Could you check a few things on this drawing? It's one solid part, dimensions in mm from its lowest x, y, z. Give positions to 0.01 mm unless a question says otherwise; leave off trailing zeros. Order: outer loops, then holes, each group sorted by start corner. A loop starts at its lowest first (then second) coordinate and runs counter-clockwise, first axis right, second up.
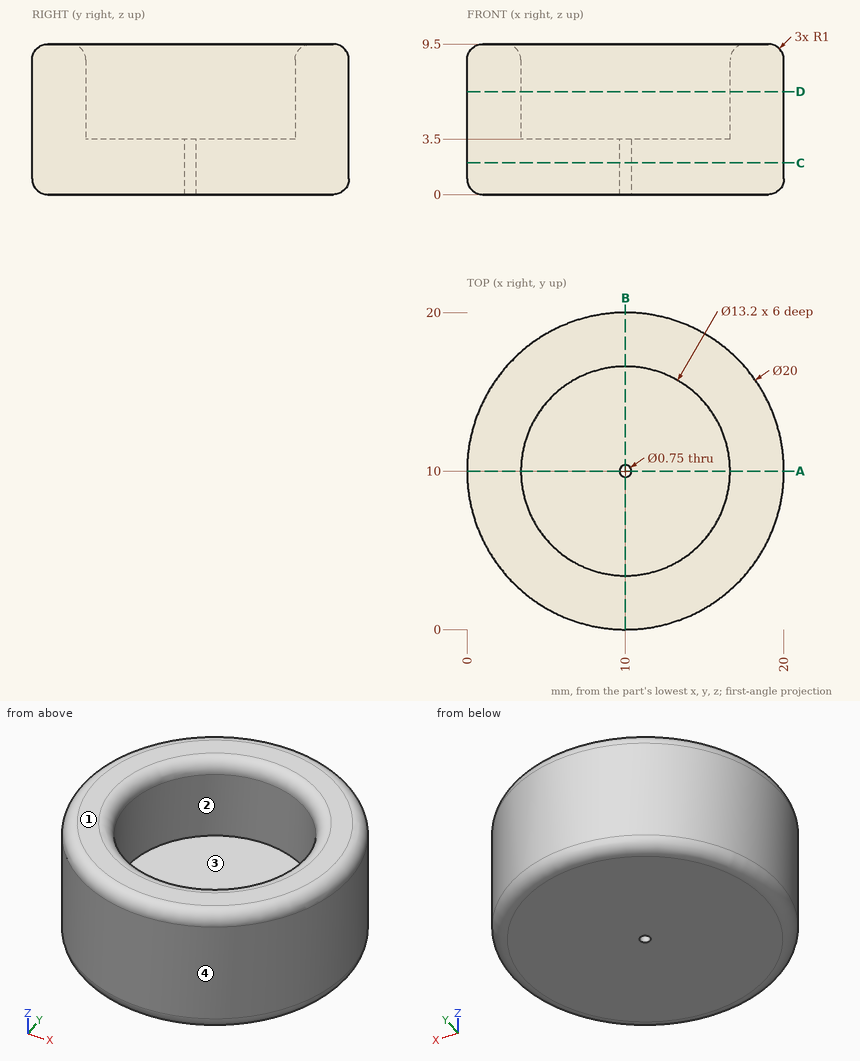
Q1. I need wall thicknesses on L1, parallel to Y at x = 10, z = 2.35 (3 decimals); L2, parallel to Y at x = 10, z = 4.9; L3, parallel to X at y = 8.5, z = 7.5. Which ranges of each line are inside material? Lowest first, please.
Filled sheet:
L1: y = 0 to 9.625, 10.375 to 20
L2: y = 0 to 3.4, 16.6 to 20
L3: x = 0.11 to 3.57, 16.43 to 19.89
Q2. If we section it at A-A on y = 10: List the corners of the cut face in (x, z) for me (3 decimals), plus the area to 3 significant figures.
Filled sheet:
outline: (0, 1) arc R1 ccw to (1, 0) - (9.625, 0) - (9.625, 3.5) - (3.4, 3.5) - (3.4, 8.5) arc R1 ccw to (2.4, 9.5) - (1, 9.5) arc R1 ccw to (0, 8.5) - close; (10.375, 0) - (19, 0) arc R1 ccw to (20, 1) - (20, 8.5) arc R1 ccw to (19, 9.5) - (17.6, 9.5) arc R1 ccw to (16.6, 8.5) - (16.6, 3.5) - (10.375, 3.5) - close
area: 107 mm2
Q3. I'm going to push flat-ended pins straight in: P1, Ø5, axis at y = 4.5, z = 4.5, coming from the -X side; P2, Ø3, axis at y = 7.5, z = 1.5, coming from the -X side; P3, Ø4, axis at x = 10.5, y = 11, coming from the +Z side. Where does each tip first touch, or does it pass through?
Filled sheet:
P1: stops at x = 0.46
P2: stops at x = 0.05
P3: stops at z = 3.5
Q4. Thinking about a two-plate mould opening in X: for the marked faces 1, 2, 3 and 4, which applies, released by +X, released by -X, zero draft, split by the parting line, or undercut?
Filled sheet:
face 1: zero draft
face 2: undercut
face 3: undercut
face 4: split by the parting line
Q5. If we section it at C-C on z = 2: List the corners of the cut face in (x, y) for me (3 decimals).
Filled sheet:
outline: circle Ø20 at (10, 10); hole circle Ø0.75 at (10, 10)
Q6. If we section it at D-D on z = 6.5: List the corners of the cut face in (x, y) for me.
Filled sheet:
outline: circle Ø20 at (10, 10); hole circle Ø13.2 at (10, 10)
